Read the model definition and answer for the solid it produces. Units are mm, in the model's axes. Face numbers are marked on the shaded views. A direction names the side the tool comes from. Give positions to 0.01 mm unless a question says otherwise; leave off trailing zeros. Order: outer loops, then holes, each group sorted by start corner. A loop starts at its lowest first (then second) coordinate and runs counter-clockwise, first axis right, second up. Notation, with made-up numbers: M 83,23.25 L 89,23.25 A17 ccw 89,45.25 Z; hole C 30,89 d3. An arc over 180 degrees is marked long. One line per item, written item: value.
from build123d import *

# Parameters (mm, degrees)
SKETCH122_R       = 3
PAD096_DEPTH      = 2.5
PAD096_DEPTH_BACK = 100
SKETCH096_R       = 1.7
PAD073_DEPTH      = 4


with BuildPart() as countersink:
    # Sketch122 → Pad096 (new body, two sides)
    with BuildSketch(Plane.XZ.offset(-26)) as pad096_sk:
        with Locations((-18.75, 0)):
            Circle(SKETCH122_R)
        with Locations((-28.75, 0)):
            Circle(SKETCH122_R)
    extrude(amount=PAD096_DEPTH)
    extrude(pad096_sk.sketch, amount=-PAD096_DEPTH_BACK)


with BuildPart() as differentialmountadapter:
    # Sketch096 → Pad073 (new body)
    with BuildSketch(Plane.XZ.offset(-20)):
        Polygon((-16.5, 7.5), (-29.490381, 15), (-34.5, 12.107695), (-31.5, 4), (-40, 2.016667), (-40, -2.016667), (-31.5, -4), (-34.5, -12.107695), (-29.490381, -15), (-16.5, -7.5), align=None)
        with Locations((-18.75, 0)):
            Circle(SKETCH096_R, mode=Mode.SUBTRACT)
        with Locations((-28.75, 0)):
            Circle(SKETCH096_R, mode=Mode.SUBTRACT)
        with Locations((-29, 10)):
            Circle(SKETCH096_R, mode=Mode.SUBTRACT)
        with Locations((-29, -10)):
            Circle(SKETCH096_R, mode=Mode.SUBTRACT)
        with Locations((-36, 0)):
            Circle(SKETCH096_R, mode=Mode.SUBTRACT)
    extrude(amount=-PAD073_DEPTH)

    # Cut007019007: cut Countersink
    add(countersink.part, mode=Mode.SUBTRACT)


with BuildPart() as part_mirroring005:
    # Part__Mirroring005: instance of DifferentialMountAdapter
    add(differentialmountadapter.part.mirror(Plane(origin=(0, 0, 0), x_dir=(0, -1, 0), z_dir=(1, 0, 0))))


solid = part_mirroring005.part
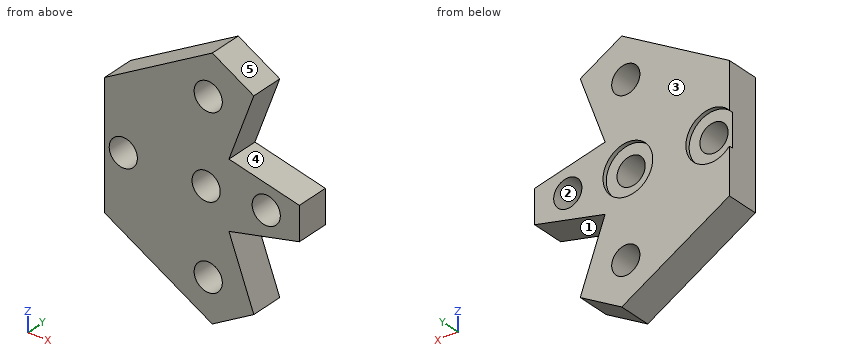
1) Which of the six approach directions +Z, -Z, +X, -X, +Y, -Y give full straight-line access (tool end or side, diameter ignored) to the marked faces 1 and 2?
Reported:
face 1: +X, +Y, -Y
face 2: +Y, -Y
2) Find section C-C, the plane y = 22.4. Write down the section's boundary in (x, z).
Reported:
outline: M 16.5,-7.5 L 29.49,-15 L 34.5,-12.11 L 31.5,-4 L 40,-2.02 L 40,2.02 L 31.5,4 L 34.5,12.11 L 29.49,15 L 16.5,7.5 Z; hole C 18.75,0 d3.4; hole C 28.75,0 d3.4; hole C 29,-10 d3.4; hole C 29,10 d3.4; hole C 36,0 d3.4
3) Find section A-A, the plane z = 0. Write down the section's boundary in (x, y).
Reported:
outline: M 16.5,20 L 17.05,20 L 17.05,23.5 L 16.5,23.5 Z; M 20.45,20 L 27.05,20 L 27.05,23.5 L 25.75,23.5 L 25.75,24 L 21.75,24 L 21.75,23.5 L 20.45,23.5 Z; M 30.45,20 L 34.3,20 L 34.3,24 L 31.75,24 L 31.75,23.5 L 30.45,23.5 Z; M 37.7,20 L 40,20 L 40,24 L 37.7,24 Z
4) This flat-tipped pin is pushed along its axis until it touches: pin 1 Ø5 at (x, z) = (28.75, 0) entering from +Y. Where does it stop, or does it pass through?
Reported:
pin 1: stops at y = 23.5
5) Determine the mould class of the marked faces 3, 4 and 5 for opening direction Z: +Z half, -Z half, draft (parallel to the pull), parting line (faces both ways), or undercut.
Reported:
face 3: draft
face 4: undercut
face 5: +Z half
6) Consider probe 1 along X at (y, z) = (20.3, 0.75); probe 2 along Z at (x, y) = (29, 21.45); probe 3 along Z at (x, y) = (29.5, 23). Determine where each line is inside the solid, lowest interval first.
Reported:
probe 1: x = 16.5 to 17.22, 20.28 to 27.22, 30.28 to 34.47, 37.53 to 40
probe 2: z = -14.72 to -11.7, -8.3 to -1.68, 1.68 to 8.3, 11.7 to 14.72
probe 3: z = -14.99 to -11.62, -8.38 to -1.53, 1.53 to 8.38, 11.62 to 14.99
7) Find section B-B, the plane x = 36. Write down the section's boundary in (y, z).
Reported:
outline: M 20,-2.95 L 24,-2.95 L 24,-1.7 L 20,-1.7 Z; M 20,1.7 L 24,1.7 L 24,2.95 L 20,2.95 Z
8) Find section D-D, the plane x = 28.75. Write down the section's boundary in (y, z), plus the area to 3 significant figures.
Reported:
outline: M 20,-14.57 L 24,-14.57 L 24,-11.68 L 20,-11.68 Z; M 20,-8.32 L 24,-8.32 L 24,-3 L 23.5,-3 L 23.5,-1.7 L 20,-1.7 Z; M 20,1.7 L 23.5,1.7 L 23.5,3 L 24,3 L 24,8.32 L 20,8.32 Z; M 20,11.68 L 24,11.68 L 24,14.57 L 20,14.57 Z
area: 74.8 mm^2
